```python
from build123d import *

# Parameters (mm, degrees)
F0_W     = 200
F0_H     = 150
F1_DEPTH = 300
F2_R     = 12
F3_T     = -5


with BuildPart() as f1:
    # F0 (on Top) → F1 (new body)
    with BuildSketch(Plane.XY):
        Rectangle(F0_W, F0_H)
    extrude(amount=F1_DEPTH)

    # F2
    f2_edges = [f1.edges().sort_by_distance(p)[0] for p in [
        (-100, 75, 150),
        (-100, 0, 300),
        (-100, -75, 150),
        (0, -75, 300),
        (100, 0, 300),
        (100, -75, 150),
        (100, 75, 150),
        (0, 75, 300),
    ]]
    fillet(f2_edges, radius=F2_R)

    # F3
    f3_openings = [f1.faces().sort_by_distance(p)[0] for p in [
        (0, 0, 0),
    ]]
    offset(amount=F3_T, openings=f3_openings)


solid = f1.part
```
Could you check a few things on this model? Use its own coordinates, in mm. A direction names the side the tool comes from. Give positions to 0.01 mm unless a question says otherwise; leave off trailing zeros. Loops run counter-clockwise (first coordinate to the right, second up) from the corner with the lowest first, then second, coordinate; pieces in that order, holes last. Notation, with made-up numbers: (-10, -4.75) - (30, -4.75) arc R7 ccw to (30, 8.25) - close; hole circle Ø7 at (11.5, 7). An arc over 180 degrees is marked (long way). Answer in a Markdown table with one row per item. Add a question column.
Q1. We'd pull the mould along X, two halves only. Please class faces 3 (the face through (93, 0.9, 292.9)), 4 (the face through (-96.58, -71.39, 146.02)), 5 (the face through (-1, -75, 142)): +X half, -X half, draft (parallel to the pull), parting line (faces both ways), or undercut.
Q2. Which directions (+Z, -Z, +X, -X, +Y, -Y) give clear straight access to the entire face, cutting with the end or side of a thin tool? Please do faces 1 (the face through (93, 67.9, 146)), 2 (the face through (100, -1, 142)).
Q3. If we section it at B-B (x = 79): List the corners of the cut face in (y, z) for me.
Q4. For pin 1 (6 mm diameter, centred on x = 9, y = 37.5, fed in from -Z), with a flat end and sliding along its axis, tell me the tip position at first contact or that it passes through.
Q5. If we section it at A-A (z = 78): List the corners of the cut face in (x, y) for me.
Q6. Please list where these lines run through material, in increasing order: L1, parallel to Y at x = 35.5, z = 182.5; L2, parallel to X at y = -63, z = 27; L3, parallel to Z at x = -22, y = 58.5. Write a range as from..to.
Q7. If we section it at C-C (y = 41.5): List the corners of the cut face in (x, z) for me.
The answers:
| question | item | result |
|---|---|---|
| 1 | face 3 | undercut |
| 1 | face 4 | -X half |
| 1 | face 5 | draft |
| 2 | face 1 | -Z |
| 2 | face 2 | +Z, -Z, +X, +Y, -Y |
| 3 | outline | (-75, 0) - (-70, 0) - (-70, 288) arc R7 cw to (-63, 295) - (63, 295) arc R7 cw to (70, 288) - (70, 0) - (75, 0) - (75, 288) arc R12 ccw to (63, 300) - (-63, 300) arc R12 ccw to (-75, 288) - close |
| 4 | pin 1 | stops at z = 295 |
| 5 | outline | (-100, -63) arc R12 ccw to (-88, -75) - (88, -75) arc R12 ccw to (100, -63) - (100, 63) arc R12 ccw to (88, 75) - (-88, 75) arc R12 ccw to (-100, 63) - close; hole (-95, -63) arc R7 ccw to (-88, -70) - (88, -70) arc R7 ccw to (95, -63) - (95, 63) arc R7 ccw to (88, 70) - (-88, 70) arc R7 ccw to (-95, 63) - close |
| 6 | L1 | y = -75..-70, 70..75 |
| 6 | L2 | x = -100..-95, 95..100 |
| 6 | L3 | z = 295..300 |
| 7 | outline | (-100, 0) - (-95, 0) - (-95, 288) arc R7 cw to (-88, 295) - (88, 295) arc R7 cw to (95, 288) - (95, 0) - (100, 0) - (100, 288) arc R12 ccw to (88, 300) - (-88, 300) arc R12 ccw to (-100, 288) - close |
